```python
from build123d import *

# Parameters (mm, degrees)
SKETCH1_W           = 57.15
SKETCH1_H           = 57.15
SKETCH1_R           = 6.99897
BOSS_EXTRUDE1_DEPTH = 3.175
SKETCH2_R           = 4.7625
CUT_EXTRUDE1_DEPTH  = 41.535686438
CIRPATTERN1_COUNT   = 4


with BuildPart() as part:
    # Sketch1 → Boss-Extrude1 (new body)
    with BuildSketch(Plane(origin=(0, 0, 0), x_dir=(0, 0, -1), z_dir=(1, 0, 0))):
        Rectangle(SKETCH1_W, SKETCH1_H)
        Circle(SKETCH1_R, mode=Mode.SUBTRACT)
    extrude(amount=BOSS_EXTRUDE1_DEPTH)

    # Sketch2 → Cut-Extrude1 (cut, through all)
    with BuildSketch(Plane(origin=(0, 0, 0), x_dir=(0, 0, -1), z_dir=(1, 0, 0))):
        with Locations((0, 19.05)):
            Circle(SKETCH2_R)
    cut_extrude1 = extrude(amount=CUT_EXTRUDE1_DEPTH, mode=Mode.SUBTRACT)

    # CirPattern1: Cut-Extrude1 ×4 about axis
    cirpattern1_axis = Axis((0, 0, 0), (1, 0, 0))
    for i in range(1, CIRPATTERN1_COUNT):
        add(cut_extrude1.rotate(cirpattern1_axis, i * 360 / CIRPATTERN1_COUNT), mode=Mode.SUBTRACT)


solid = part.part
```
For this review, take the finished solid that the model builds, in its own axes (mm). Give positions to 0.01 mm unless a question says otherwise; leave off trailing zeros. Write each loop counter-clockwise with the first axis right and the second up, starting at its lowest first coordinate (ties: lowest second). Pieces come first, ordered by that corner, then holes. Notation, with made-up numbers: M 35.25,37 L 81.25,37 A15 ccw 81.25,66 Z; hole C 0,12 d8. An arc over 180 degrees is marked long. One line per item, written item: value.
1) For line 1 (Y direction, x = 1.1, z = 0) (1 decimal); line 2 (Y direction, x = 1.05, z = -19.05) (1 decimal); line 3 (Z direction, x = 2.25, y = -19) (3 decimals), list the stretches that pass through material, from the lowest coordinate up. Write a range as from..to.
Results are:
line 1: y = -28.6..-23.8, -14.3..-7, 7..14.3, 23.8..28.6
line 2: y = -28.6..-4.8, 4.8..28.6
line 3: z = -28.575..-4.762, 4.762..28.575
2) Take a section at C-C, the plane x = 1.8. Count the separate pieces of the cut face and the enclosed holes in it, then the cut area to 3 significant figures.
Results are:
separate pieces: 1
enclosed holes: 5
area: 2,830 mm²
3) Take a section at D-D, the plane z = 0. Write out the cut boundary in (x, y) (1 decimal), then the cut area to 3 significant figures.
Results are:
outline: M 0,-28.6 L 3.2,-28.6 L 3.2,-23.8 L 0,-23.8 Z; M 0,-14.3 L 3.2,-14.3 L 3.2,-7 L 0,-7 Z; M 0,7 L 3.2,7 L 3.2,14.3 L 0,14.3 Z; M 0,23.8 L 3.2,23.8 L 3.2,28.6 L 0,28.6 Z
area: 76.5 mm²
4) The part is to be moulded in two halves that separate along Z. For faces 1 (the cylindrical face through (1.57, -6.83, 1.52)), 2 (the flat face through (2, 0, 28.575)), 3 (the flat face through (2, 28.575, 0)), say which applies: +Z half, -Z half, draft (parallel to the pull), parting line (faces both ways), or undercut.
Results are:
face 1: undercut
face 2: +Z half
face 3: draft
5) Take a section at A-A, the plane z = -19.05. Write out the cut boundary in (x, y) (1 decimal), then the cut area to 3 significant figures.
Results are:
outline: M 0,-28.6 L 3.2,-28.6 L 3.2,-4.8 L 0,-4.8 Z; M 0,4.8 L 3.2,4.8 L 3.2,28.6 L 0,28.6 Z
area: 151 mm²
